from build123d import *

# Parameters (mm, degrees)
SKETCH1_W           = 838.2
SKETCH1_H           = 673.1
BOSS_EXTRUDE1_DEPTH = 19.05
CHAMFER1_SIZE       = 2.54
CHAMFER2_SIZE       = 2.54
SKETCH2_R           = 3.175
CUT_EXTRUDE1_DEPTH  = 20.05


with BuildPart() as part:
    # Sketch1 → Boss-Extrude1 (new body)
    with BuildSketch(Plane(origin=(0, 0, 0), x_dir=(1, 0, 0), z_dir=(0, 1, 0))):
        with Locations((419.1, 336.55)):
            Rectangle(SKETCH1_W, SKETCH1_H)
    extrude(amount=BOSS_EXTRUDE1_DEPTH)

    # Chamfer1
    chamfer1_edges = [part.edges().sort_by_distance(p)[0] for p in [
        (838.2, 19.05, -336.55),
        (419.1, 19.05, -673.1),
        (0, 19.05, -336.55),
        (419.1, 19.05, 0),
    ]]
    chamfer(chamfer1_edges, length=CHAMFER1_SIZE)

    # Chamfer2
    chamfer2_edges = [part.edges().sort_by_distance(p)[0] for p in [
        (419.1, 0, -673.1),
    ]]
    chamfer(chamfer2_edges, length=CHAMFER2_SIZE)

    # Sketch2 → Cut-Extrude1 (cut, through all)
    with BuildSketch(Plane(origin=(0, 19.05, 0), x_dir=(1, 0, 0), z_dir=(0, 1, 0))):
        with Locations((101.6, 542.925)):
            Circle(SKETCH2_R)
        with Locations((101.6, 203.2)):
            Circle(SKETCH2_R)
        with Locations((711.2, 542.925)):
            Circle(SKETCH2_R)
        with Locations((711.2, 203.2)):
            Circle(SKETCH2_R)
    extrude(amount=-CUT_EXTRUDE1_DEPTH, mode=Mode.SUBTRACT)


solid = part.part
The listing builds one solid part. Answer for the finished solid, in the listing's coordinates (mm). Give positions to 0.01 mm unless a question says otherwise; leave off trailing zeros. Use one line per item in the form item = value.
1. Given pin 1 Ø2 at (x, z) = (181, -67.5) entering from -Y; pin 2 Ø5 at (x, z) = (101.6, -203.2) entering from +Y, each flat-ended and moving along its own axis, determine where each tip first touches the part or whether it passes through.
Calculated:
pin_1 = 0
pin_2 = through
2. Find the intervals of material crossed by line 1 along Z through (x, y) = (711.2, 10) (3 decimals); line 2 along X through (y, z) = (5, -203.2) (3 decimals); line 3 along X through (y, z) = (17.75, -180.5), in increasing order. Write a range as [from, to].
Calculated:
line_1 = [-673.1, -546.1], [-539.75, -206.375], [-200.025, 0]
line_2 = [0, 98.425], [104.775, 708.025], [714.375, 838.2]
line_3 = [1.24, 836.96]
3. The mould has two halves that part along X. Classify faces 1 (the face through (413, 0, -340)), 2 (the face through (838.2, 8, -332)), 3 (the face through (0, 8, -332)): pulls with the +X half, pulls with the -X half, needs draft (parallel to the pull), parting line crosses it, or undercut.
Calculated:
face_1 = needs draft
face_2 = pulls with the +X half
face_3 = pulls with the -X half
